Autodesk Inventor part; units mm, degrees
ref_plane "YZ Plane" through (0, 0, 0) normal (1, 0, 0) x (0, 1, 0)
ref_plane "XZ Plane" through (0, 0, 0) normal (0, 1, 0) x (-1, 0, 0)
ref_plane "XY Plane" through (0, 0, 0) normal (0, 0, 1) x (1, 0, 0)
sketch "Sketch1" plane through (0, 0, 0) normal (0, 0, 1) x (1, 0, 0)
  circle A0 centre (0, 39) radius 1.5
  circle A1 centre (29, 39) radius 1.5
  line L0 (-2.5, 36.5) -> (2.5, 36.5)
  line L1 (2.5, 36.5) -> (2.5, 39.5)
  line L2 (2.5, 39.5) -> (26.5, 39.5)
  line L3 (26.5, 39.5) -> (26.5, 36.5)
  line L4 (26.5, 36.5) -> (31.5, 36.5)
  line L5 (31.5, 36.5) -> (31.5, 39.5)
  arc A2 (31.5, 39.5) -> (27.5, 43.5) centre (27.5, 39.5) ccw
  line L6 (27.5, 43.5) -> (-2.5, 43.5)
  line L7 (-2.5, 43.5) -> (-2.5, 36.5)
  point P0 (0, 0)
extrude "Extrusion1" add sketch "Sketch1" along normal blind 6
properties part number "yCarMid_b"
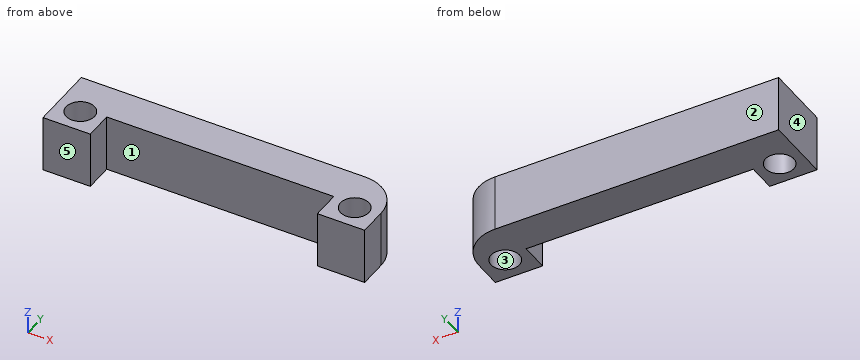
Geometry: final body of the model. Coordinates: model frame, mm. Face numbers are marked on the shaded views. A direction names the side the tool comes from. Coordinates: 2 decimals unless noted, no trailing zeros. Write each loop counter-clockwise with the first axis right and the second up, starting at its lowest first coordinate (ties: lowest second). Pieces come first, ordered by that corner, then holes. Notation, with made-up numbers: M 78.5,-7 L 88.5,-7 A26 cw 88.5,32 Z; hole C -12,13.25 d5. An arc over 180 degrees is marked long. Answer as CSV lines item,"result". Start each with the question number.
Q1. Reachability of the marked faces 1 and 2 from +Z, -Z, +X, -X, +Y, -Y: full face, straight path, thin tool, end or side. Return the list, or none.
Q2. Pin query (flat end, axial travel): P1, Ø2, axis at y = 41.5, z = 1.5, coming from the +X side; P2, Ø1.8, axis at x = 13.5, z = 4.5, coming from the -Y side. Return the tip coordinate at first contact, or that it passes through.
Q3. Line query: line 1 (Y direction, x = 0, z = 1.3); line 2 (X direction, y = 38.5, z = 2.7); line 3 (X direction, y = 38.25, z = 0.3). Output: solid intervals per line, ascending. Write a range as from..to.
Q4. Cut plane B-B on x = 0. Return the cut outline in (y, z).
Q5. Cut plane C-C on y = 38.5. Return the cut outline in (x, z), then the cut area to 3 significant figures.
Q6. Cut plane A-A on z = 2.55. Return the cut outline in (x, y).
Q7. Mould query, pull axis X, two halves, no side actions, for the marked faces 3, 4 and 5. Classes: released by +X, released by -X, zero draft, split by the parting line, or undercut.
Q8. Cut plane D-D on x = 29. Return the cut outline in (y, z), then the cut area to 3 significant figures.
Findings below:
1,face 1,"+Z, -Z, -Y"
1,face 2,"+Z, -Z, +X, -X, +Y"
2,P1,"stops at x = 31.37"
2,P2,"stops at y = 39.5"
3,line 1,"y = 36.5..37.5, 40.5..43.5"
3,line 2,"x = -2.5..-1.41, 1.41..2.5, 26.5..27.59, 30.41..31.5"
3,line 3,"x = -2.5..-1.3, 1.3..2.5, 26.5..27.7, 30.3..31.5"
4,outline,"M 36.5,0 L 37.5,0 L 37.5,6 L 36.5,6 Z; M 40.5,0 L 43.5,0 L 43.5,6 L 40.5,6 Z"
5,outline,"M -2.5,0 L -1.41,0 L -1.41,6 L -2.5,6 Z; M 1.41,0 L 2.5,0 L 2.5,6 L 1.41,6 Z; M 26.5,0 L 27.59,0 L 27.59,6 L 26.5,6 Z; M 30.41,0 L 31.5,0 L 31.5,6 L 30.41,6 Z"
5,area,"26.1 mm2"
6,outline,"M -2.5,36.5 L 2.5,36.5 L 2.5,39.5 L 26.5,39.5 L 26.5,36.5 L 31.5,36.5 L 31.5,39.5 A4 ccw 27.5,43.5 L -2.5,43.5 Z; hole C 0,39 d3; hole C 29,39 d3"
7,face 3,"undercut"
7,face 4,"released by -X"
7,face 5,"zero draft"
8,outline,"M 36.5,0 L 37.5,0 L 37.5,6 L 36.5,6 Z; M 40.5,0 L 43.21,0 L 43.21,6 L 40.5,6 Z"
8,area,"22.2 mm2"
